Autodesk Inventor part; units mm, degrees
ref_plane "YZ Plane" through (0, 0, 0) normal (1, 0, 0) x (0, 1, 0)
ref_plane "XZ Plane" through (0, 0, 0) normal (0, 1, 0) x (-1, 0, 0)
ref_plane "XY Plane" through (0, 0, 0) normal (0, 0, 1) x (1, 0, 0)
sketch "Boceto2" plane through (0, 0, 0) normal (0, 1, 0) x (-1, 0, 0)
  line L0 (7.5, 100) -> (-7.5, 100)
  line L1 (-7.5, 100) -> (-7.5, -100)
  line L2 (-7.5, -100) -> (7.5, -100)
  line L3 (7.5, -100) -> (7.5, 100)
  line L4 (7.5, 100) -> (-7.5, -100) construction
  line L5 (-7.5, 100) -> (7.5, -100) construction
  point P0 (0, 0)
  dimension "d7" = 15
  dimension "d8" = 200
extrude "Extrusión1" add sketch "Boceto2" along normal blind 10
sketch "Boceto3" plane through (0, 10, 0) normal (0, 1, 0) x (1, 0, 0)
  line L0 (5, 60) -> (-5, 60)
  line L1 (-5, 60) -> (-5, 70)
  line L2 (-5, 70) -> (5, 70)
  line L3 (5, 70) -> (5, 60)
  line L4 (5, 60) -> (-5, 70) construction
  line L5 (7.5, 100) -> (-7.5, 100)
  line L6 (0, 64.5148) -> (0, 61.9205)
  circle A0 centre (3.25, 61.75) radius 1.75
  circle A1 centre (-3.25, 68.25) radius 1.75
  line L7 (-7.5, 100) -> (-7.5, -100)
  line L8 (-7.5, 0) -> (0, 0)
  line L9 (5, -70) -> (5, -60)
  line L10 (-5, -70) -> (5, -70)
  line L11 (5, -60) -> (-5, -60)
  line L12 (-5, -60) -> (-5, -70)
  line L13 (5, -60) -> (-5, -70) construction
  line L14 (0, -64.5148) -> (0, -61.9205)
  circle A2 centre (-3.25, -68.25) radius 1.75
  circle A3 centre (3.25, -61.75) radius 1.75
  point P0 (3.25, 68.25)
  point P1 (-5, 65)
  point P2 (-3.25, 61.75)
  point P3 (0, 100)
  point P4 (3.25, -68.25)
  point P5 (-3.25, -61.75)
  point P6 (-5, -65)
  dimension "d12" = 1.75
  dimension "d13" = 1.75
  dimension "d14" = 1.75
  dimension "d15" = 1.75
  dimension "d16" = 10
  dimension "d17" = 10
  dimension "d19" = 30
  dimension "d67" = 31.75
hole "Agujero1" at (3.25, 10, -61.75) at (-3.25, 10, -68.25) at (-3.25, 10, 68.25) at (3.25, 10, 61.75) direction (0, -1, 0) diameter 3.5 end through all
sketch "Boceto4" plane through (0, 10, 0) normal (0, 1, 0) x (1, 0, 0)
  line L0 (-7.5, 100) -> (-7.5, -100)
  line L1 (-7.5, -100) -> (7.5, -100)
  line L2 (7.5, -100) -> (7.5, -80)
  line L3 (7.5, -80) -> (-7.5, -80)
  line L4 (-7.5, -80) -> (-7.5, -100)
  line L5 (-7.5, 0) -> (1.0116, 0)
  line L6 (-7.5, -100) -> (-7.5, 100)
  line L7 (-7.5, 100) -> (7.5, 100)
  line L8 (7.5, 100) -> (7.5, 80)
  line L9 (7.5, 80) -> (-7.5, 80)
  line L10 (-7.5, 80) -> (-7.5, 100)
  point P0 (0, 0)
  point P1 (-7.5, -80)
  point P2 (-7.5, 80)
  dimension "d27" = 15
  dimension "d28" = 20
extrude "Extrusión2" add sketch "Boceto4" along normal blind 80
sketch "Boceto5" plane through (0, 90, 0) normal (0, 1, 0) x (1, 0, 0)
  line L0 (-7.5, -100) -> (7.5, -100)
  line L1 (-7.5, -100) -> (40.5, -100)
  line L2 (40.5, -100) -> (40.5, 100)
  line L3 (40.5, 100) -> (-7.5, 100)
  line L4 (-7.5, 100) -> (-7.5, -100)
  line L5 (40.5, -100) -> (-159.5, -100)
  line L6 (-159.5, -100) -> (-159.5, 100)
  line L7 (-159.5, 100) -> (40.5, 100)
  line L8 (40.5, 100) -> (40.5, -100)
  point P0 (0, 0)
  point P1 (-7.5, 100)
  dimension "d31" = 48
  dimension "d32" = 200
  dimension "d74" = 200
extrude "Extrusión3" add sketch "Boceto5" along normal blind 110
sketch "Boceto6" plane through (0, 200, 0) normal (0, 1, 0) x (1, 0, 0)
  line L0 (40.5, 100) -> (7.5, 100)
  line L1 (40.5, 100) -> (20.5, 100)
  line L2 (20.5, 100) -> (20.5, 80)
  line L3 (7.5, -100) -> (40.5, -100)
  line L4 (24, -100) -> (24, -80)
  line L5 (-159.5, 100) -> (-159.5, -100)
  line L6 (20.5, 80) -> (-159.5, 80)
  line L7 (-159.5, 80) -> (-159.5, -80)
  line L8 (-159.5, -80) -> (20.5, -80)
  line L9 (20.5, -80) -> (20.5, 80)
  line L10 (-159.5, -100) -> (40.5, -100)
  point P0 (7.5, 80)
  point P1 (-159.5, 80)
  dimension "d36" = 20
  dimension "d37" = 20
  dimension "d38" = 20
  dimension "d78" = 20
extrude "Extrusión4" cut sketch "Boceto6" against normal blind 90
sketch "Boceto7" plane through (-159.5, 90, -100) normal (-1, 0, 0) x (0, 0, 1)
  line L0 (0, 110) -> (20, 110)
  line L1 (20, 110) -> (10, 110)
  line L2 (10, 110) -> (10, 20)
  line L3 (10, 20) -> (20, 20)
  line L4 (20, 20) -> (20, 110)
  line L5 (180, 110) -> (180, 20)
  line L6 (180, 110) -> (190, 110)
  line L7 (190, 110) -> (190, 20)
  line L8 (190, 20) -> (180, 20)
  line L9 (180, 20) -> (180, 110)
  line L10 (200, 0) -> (200, 110)
  line L11 (0, 0) -> (0, 110)
  line L12 (0, 110) -> (10, 110)
  line L13 (10, 110) -> (10, 20)
  line L14 (10, 20) -> (0, 20)
  line L15 (0, 20) -> (0, 110)
  line L16 (200, 110) -> (0, 110)
  line L17 (200, 110) -> (190, 110)
  line L18 (190, 110) -> (190, 20)
  line L19 (190, 20) -> (200, 20)
  line L20 (200, 20) -> (200, 110)
  point P0 (100, -90)
  point P1 (200, 20)
  dimension "d42" = 10
  dimension "d63" = 10
  dimension "d65" = 10
extrude "Extrusión5" cut sketch "Boceto7" against normal blind 30 contours L0 L2 L14 L11 | L16 L10 L19 L7
sketch "Boceto8" plane through (-7.5, 0, 100) normal (0, 0, 1) x (1, 0, 0)
  line L0 (-122, 200) -> (-122, 110)
  line L1 (-132, 175) -> (-142, 175)
  line L2 (-142, 175) -> (-142, 185)
  line L3 (-142, 185) -> (-132, 185)
  line L4 (-132, 185) -> (-132, 175)
  line L5 (-132, 175) -> (-142, 185) construction
  line L6 (-142, 175) -> (-132, 185) construction
  line L7 (-152, 200) -> (48, 200)
  line L8 (-113, 155) -> (-128, 155)
  line L9 (-152, 110) -> (-122, 110)
  line L10 (-132, 180) -> (-131.5898, 180)
  circle A0 centre (-140.25, 183.25) radius 1.75
  circle A1 centre (-133.75, 176.75) radius 1.75
  line L11 (-132, 125) -> (-132, 135)
  line L12 (-142, 125) -> (-132, 125)
  line L13 (-132, 135) -> (-142, 125) construction
  line L14 (-132, 135) -> (-142, 135)
  line L15 (-142, 135) -> (-132, 125) construction
  line L16 (-142, 135) -> (-142, 125)
  line L17 (-132, 130) -> (-131.5898, 130)
  circle A2 centre (-133.75, 133.25) radius 1.75
  circle A3 centre (-140.25, 126.75) radius 1.75
  line L18 (-152, 110) -> (-152, 200)
  point P0 (7.5, 0)
  point P1 (-113, 215)
  point P2 (-133.75, 183.25)
  point P3 (-142, 180)
  point P4 (-140.25, 176.75)
  point P5 (48, 200)
  point P6 (-133.75, 126.75)
  point P7 (-140.25, 133.25)
  point P8 (-143, 115)
  point P9 (-133.75, 126.75)
  point P10 (-140.25, 133.25)
  point P11 (-142, 130)
  dimension "d46" = 1.75
  dimension "d47" = 1.75
  dimension "d48" = 1.75
  dimension "d49" = 1.75
  dimension "d50" = 10
  dimension "d51" = 10
  dimension "d52" = 15
  dimension "d66" = 10
  dimension "d70" = 15
hole "Agujero2" at (-147.75, 183.25, 100) at (-141.25, 176.75, 100) at (-147.75, 126.75, 100) at (-141.25, 133.25, 100) direction (0, 0, -1) diameter 3.5 end through all
properties part number "container_back"
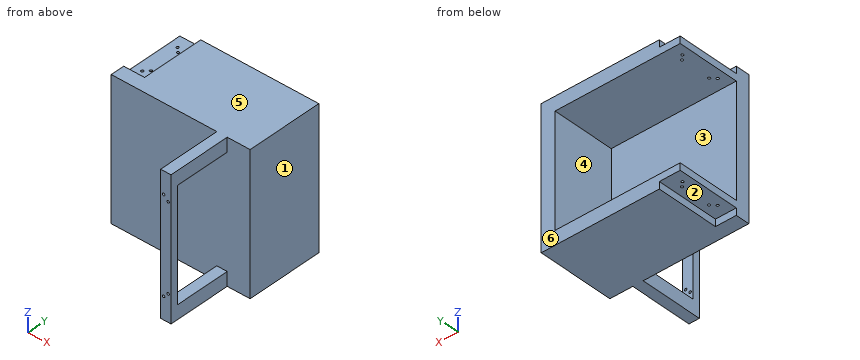
Geometry check sheet. Reference: the model listing, model coordinates, mm. Face numbers are marked on the shaded views. A direction names the side the tool comes from. Round coordinates to 2 decimals unless told otherwise and drop trailing zeros. Order: outer loops, then holes, each group sorted by start corner. A loop starts at its lowest first (then second) coordinate and runs counter-clockwise, first axis right, second up. Notation, with made-up numbers: (24.5, 29.25) - (38.5, 29.25) arc R21 cw to (38.5, 48.25) - close; hole circle Ø11 at (87, 1.5). An arc over 180 degrees is marked (long way). One line per question, with ' | ' between items. Start each with the question number.
(1) Release check for a two-part mould opening along Z. For the marked faces 4, 5 and 6 record: released by +Z, released by -Z, zero draft, split by the parting line, or undercut.
(2) Access from +Z, -Z, +X, -X, +Y, -Y to the whole of each face (thin tool, end or side, straight path). Record for the marked faces 1, 2 and 3.
(3) Sectioned sample at A-A on z = -86. Record the cut outline in (x, y), and give its area (3 significant figures).
(4) Sectioned sample at D-D on z = -46. Record the cut outline in (x, y).
(5) Depth check by flat-ended pin: pin 1 Ø2 at (x, y) = (-147.75, 126.75) entering from +Z; pin 2 Ø4.5 at (x, z) = (-1.5, 32.5) entering from +Y; pin 3 Ø5 at (y, z) = (152, 97) entering from -X; pin 4 Ø4 at (x, y) = (-147.75, 183.25) entering from -Z. Enter the tip coordinate at first touch or a pass-through.
(6) Sectioned sample at C-C on x = -135. Record the cut outline in (y, z).
(7) Thickness scan on L1, parallel to Z at x = -3.25, y = 7.5; L2, parallel to Y at x = -141.25, z = -84; L3, parallel to Y at x = -147, z = -84. Record the ranges inside material, lowest first. Write a range as [from, to].
(8) Sectioned sample at B-B on y = 34. Record the cut outline in (x, z).
Conclusion:
1) face 4: undercut | face 5: released by +Z | face 6: zero draft
2) face 1: +Z, -Z, +X, +Y, -Y | face 2: -Z, -X, +Y | face 3: -X, +Y
3) outline: (-159.5, 90) - (-7.5, 90) - (-7.5, 0) - (7.5, 0) - (7.5, 90) - (40.5, 90) - (40.5, 200) - (-159.5, 200) - close; hole circle Ø3.5 at (-147.75, 126.75); hole circle Ø3.5 at (-147.75, 183.25); hole circle Ø3.5 at (-141.25, 133.25); hole circle Ø3.5 at (-141.25, 176.75) | area: 23,300 mm2
4) outline: (-159.5, 90) - (40.5, 90) - (40.5, 200) - (20.5, 200) - (20.5, 110) - (-159.5, 110) - close; (-7.5, 0) - (7.5, 0) - (7.5, 10) - (-7.5, 10) - close
5) pin 1: passes through | pin 2: stops at y = 110 | pin 3: stops at x = -129.5 | pin 4: stops at z = -90
6) outline: (90, -100) - (110, -100) - (110, -90) - (200, -90) - (200, -80) - (110, -80) - (110, 80) - (200, 80) - (200, 90) - (110, 90) - (110, 100) - (90, 100) - close
7) L1: z = [-100, -70], [-66.5, 66.5], [70, 100] | L2: y = [90, 131.5], [135, 175], [178.5, 200] | L3: y = [90, 125.17], [128.33, 181.67], [184.83, 200]
8) outline: (-7.5, -100) - (7.5, -100) - (7.5, -80) - (-7.5, -80) - close; (-7.5, 80) - (7.5, 80) - (7.5, 100) - (-7.5, 100) - close
